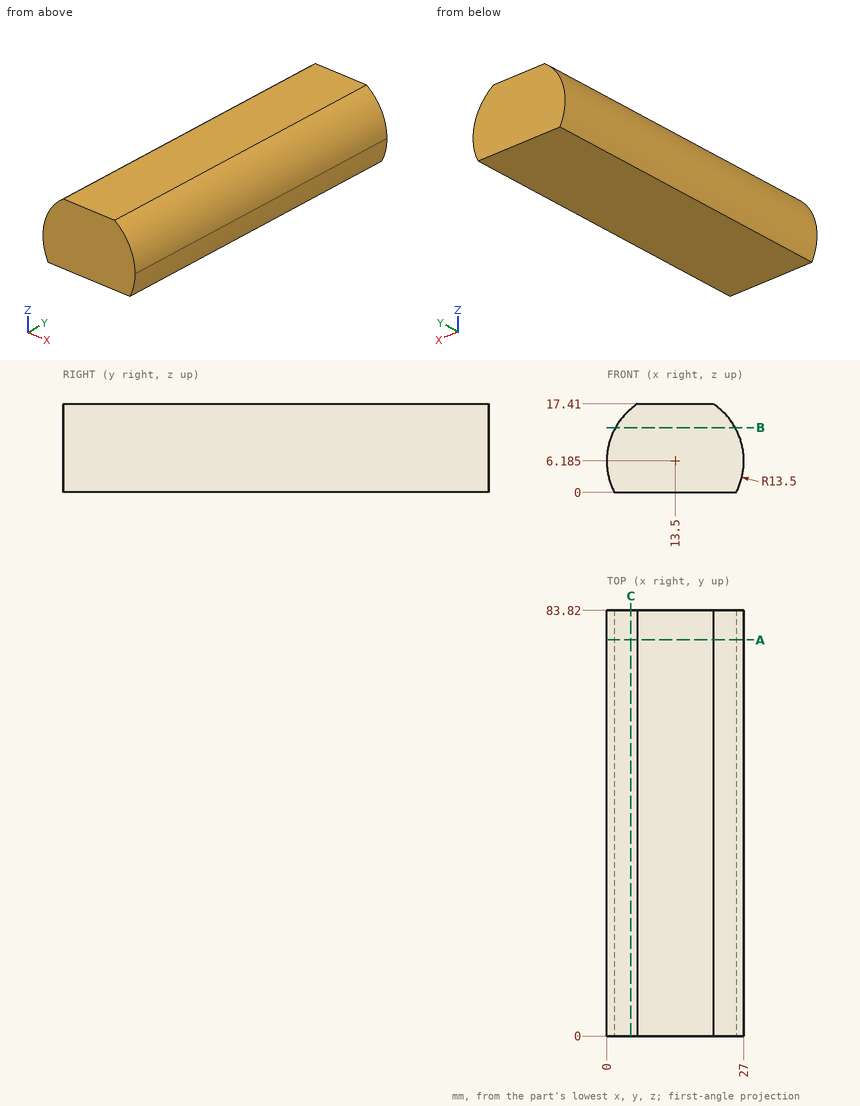
For this review, use the dimensioned drawing (mm, ordinates from the lowest corner) and the shaded views. Give positions to 0.01 mm unless a question says otherwise; leave off trailing zeros. Order: outer loops, then holes, each group sorted by start corner. A loop starts at its lowest first (then second) coordinate and runs counter-clockwise, first axis right, second up.
1) Take a section at B-B (z = 12.75). Give the boundary of the cut face in (x, y), then the cut area to 3 significant figures.
2) Take a section at A-A (y = 78). Give the boundary of the cut face in (x, z) (1 decimal).
3) Take a section at C-C (x = 4.75). Give the boundary of the cut face in (y, z) (1 decimal), then the cut area to 3 significant figures.
4) Insertion check: pin 1 (5 mm diameter, centred on y = 50.5, z = 3, fed in from -X); pin 2 (1 mm diameter, centred on y = 46.5, z = 7, fed in from +X); pin 3 (6 mm diameter, centred on y = 70, z = 11.5, fed in from +X). Each pin has a flat end and moves straight along its axis. Give the tip position at first contact, or say it passes through.
5) Wall thickness on line 1 (X direction, y = 76.5, z = 5.5); line 2 (X direction, y = 70.5, z = 7.5) (1 decimal); line 3 (Z direction, x = 23, y = 37) (1 decimal): over which ranges is each line inside the solid? List them lowest first.
Derived:
1. outline: (1.7, 0) - (25.3, 0) - (25.3, 83.82) - (1.7, 83.82) - close
1. area: 1,980 mm2
2. outline: (1.5, 0) - (25.5, 0) arc R13.5 ccw to (27, 6.2) arc R13.5 ccw to (21, 17.4) - (6, 17.4) arc R13.5 ccw to start
3. outline: (0, 0) - (83.8, 0) - (83.8, 16.5) - (0, 16.5) - close
3. area: 1,380 mm2
4. pin 1: stops at x = 0.02
4. pin 2: stops at x = 27
4. pin 3: stops at x = 26.8
5. line 1: x = 0.02 to 26.98
5. line 2: x = 0.1 to 26.9
5. line 3: z = 0 to 15.8
